```python
from build123d import *

# Parameters (mm, degrees)
SKETCH1_W           = 70.3
SKETCH1_H           = 128.3
BOSS_EXTRUDE1_DEPTH = 27.5
FILLET1_R           = 10
CUT_EXTRUDE1_START  = 35.15
CUT_EXTRUDE1_DEPTH  = 0.5
CUT_EXTRUDE2_DEPTH  = 0.5
FILLET2_R           = 10
CUT_EXTRUDE3_DEPTH  = 0.25


with BuildPart() as part:
    # Sketch1 → Boss-Extrude1 (new body)
    with BuildSketch(Plane(origin=(0, 0, 0), x_dir=(1, 0, 0), z_dir=(0, 1, 0))):
        Rectangle(SKETCH1_W, SKETCH1_H)
    extrude(amount=BOSS_EXTRUDE1_DEPTH)

    # Fillet1
    fillet1_edges = [part.edges().sort_by_distance(p)[0] for p in [
        (-35.15, 27.5, 0),
        (0, 27.5, 64.15),
        (35.15, 27.5, 0),
        (0, 0, 64.15),
        (-35.15, 0, 0),
        (0, 0, -64.15),
        (35.15, 0, 0),
        (0, 27.5, -64.15),
    ]]
    fillet(fillet1_edges, radius=FILLET1_R)

    # Sketch2 → Cut-Extrude1 (cut)
    with BuildSketch(Plane(origin=(0, 0, 0), x_dir=(0, 0, -1), z_dir=(1, 0, 0)).offset(CUT_EXTRUDE1_START)):
        with BuildLine():
            Line((48, 16.4), (53, 16.4))
            ThreePointArc((53, 16.4), (55.65, 13.75), (53, 11.1))
            Line((53, 11.1), (48, 11.1))
            ThreePointArc((48, 11.1), (45.35, 13.75), (48, 16.4))
        make_face()
        with BuildLine():
            Line((48, 15.9), (53, 15.9))
            ThreePointArc((53, 15.9), (55.15, 13.75), (53, 11.6))
            Line((53, 11.6), (48, 11.6))
            ThreePointArc((48, 11.6), (45.85, 13.75), (48, 15.9))
        make_face(mode=Mode.SUBTRACT)
    extrude(amount=-CUT_EXTRUDE1_DEPTH, mode=Mode.SUBTRACT)

    # Sketch3 → Cut-Extrude2 (cut)
    with BuildSketch(Plane(origin=(0, 27.5, 0), x_dir=(1, 0, 0), z_dir=(0, 1, 0))):
        with BuildLine():
            Line((11.275, 54.65), (20.275, 54.65))
            ThreePointArc((20.275, 54.65), (25.15, 49.775), (20.275, 44.9))
            Line((20.275, 44.9), (11.275, 44.9))
            ThreePointArc((11.275, 44.9), (6.4, 49.775), (11.275, 54.65))
        make_face()
        with BuildLine():
            Line((11.275, 54.15), (20.275, 54.15))
            ThreePointArc((20.275, 54.15), (24.65, 49.775), (20.275, 45.4))
            Line((20.275, 45.4), (11.275, 45.4))
            ThreePointArc((11.275, 45.4), (6.9, 49.775), (11.275, 54.15))
        make_face(mode=Mode.SUBTRACT)
    extrude(amount=-CUT_EXTRUDE2_DEPTH, mode=Mode.SUBTRACT)

    # Fillet2
    # the kernel refuses this fillet: 10 mm, written as the material it takes off along each edge
    with BuildSketch(Plane(origin=(25.15, 10, 54.15), x_dir=(0, 0, 1), z_dir=(1, 0, 0))) as fillet2_piece_1_section:
        Polygon((0, 0), (FILLET2_R * 1.02, 0), (FILLET2_R * 1.02, FILLET2_R * 1.02), (0, FILLET2_R * 1.02), align=None)
    fillet2_piece_1 = extrude(amount=FILLET2_R * 1.02, mode=Mode.PRIVATE)
    fillet2_piece_1 = fillet2_piece_1 - Plane(origin=(25.15, 10, 54.15), x_dir=(0, 0.7071067811865475, -0.7071067811865475), z_dir=(1, 0, 0)) * Sphere(FILLET2_R, mode=Mode.PRIVATE)
    add(fillet2_piece_1, mode=Mode.SUBTRACT)
    with BuildSketch(Plane(origin=(-25.15, 10, 54.15), x_dir=(0, 0, 1), z_dir=(-1, 0, 0))) as fillet2_piece_2_section:
        Polygon((0, 0), (FILLET2_R * 1.02, 0), (FILLET2_R * 1.02, -FILLET2_R * 1.02), (0, -FILLET2_R * 1.02), align=None)
    fillet2_piece_2 = extrude(amount=FILLET2_R * 1.02, mode=Mode.PRIVATE)
    fillet2_piece_2 = fillet2_piece_2 - Plane(origin=(-25.15, 10, 54.15), x_dir=(0, 0.7071067811865475, -0.7071067811865475), z_dir=(-1, 0, 0)) * Sphere(FILLET2_R, mode=Mode.PRIVATE)
    add(fillet2_piece_2, mode=Mode.SUBTRACT)
    with BuildSketch(Plane(origin=(25.15, 10, -54.15), x_dir=(1, 0, 0), z_dir=(0, 0, -1))) as fillet2_piece_3_section:
        Polygon((0, 0), (FILLET2_R * 1.02, 0), (FILLET2_R * 1.02, FILLET2_R * 1.02), (0, FILLET2_R * 1.02), align=None)
    fillet2_piece_3 = extrude(amount=FILLET2_R * 1.02, mode=Mode.PRIVATE)
    fillet2_piece_3 = fillet2_piece_3 - Plane(origin=(25.15, 10, -54.15), x_dir=(-0.7071067811865475, 0.7071067811865475, 0), z_dir=(0, 0, -1)) * Sphere(FILLET2_R, mode=Mode.PRIVATE)
    add(fillet2_piece_3, mode=Mode.SUBTRACT)
    with BuildSketch(Plane(origin=(-25.15, 10, -54.15), x_dir=(-1, 0, 0), z_dir=(0, 0, -1))) as fillet2_piece_4_section:
        Polygon((0, 0), (FILLET2_R * 1.02, 0), (FILLET2_R * 1.02, -FILLET2_R * 1.02), (0, -FILLET2_R * 1.02), align=None)
    fillet2_piece_4 = extrude(amount=FILLET2_R * 1.02, mode=Mode.PRIVATE)
    fillet2_piece_4 = fillet2_piece_4 - Plane(origin=(-25.15, 10, -54.15), x_dir=(0.7071067811865475, 0.7071067811865475, 0), z_dir=(0, 0, -1)) * Sphere(FILLET2_R, mode=Mode.PRIVATE)
    add(fillet2_piece_4, mode=Mode.SUBTRACT)
    with BuildSketch(Plane(origin=(-25.15, 17.5, -54.15), x_dir=(-1, 0, 0), z_dir=(0, 0, -1))) as fillet2_piece_5_section:
        Polygon((0, 0), (FILLET2_R * 1.02, 0), (FILLET2_R * 1.02, FILLET2_R * 1.02), (0, FILLET2_R * 1.02), align=None)
    fillet2_piece_5 = extrude(amount=FILLET2_R * 1.02, mode=Mode.PRIVATE)
    fillet2_piece_5 = fillet2_piece_5 - Plane(origin=(-25.15, 17.5, -54.15), x_dir=(0.7071067811865475, -0.7071067811865475, 0), z_dir=(0, 0, -1)) * Sphere(FILLET2_R, mode=Mode.PRIVATE)
    add(fillet2_piece_5, mode=Mode.SUBTRACT)
    with BuildSketch(Plane(origin=(25.15, 17.5, -54.15), x_dir=(1, 0, 0), z_dir=(0, 0, -1))) as fillet2_piece_6_section:
        Polygon((0, 0), (FILLET2_R * 1.02, 0), (FILLET2_R * 1.02, -FILLET2_R * 1.02), (0, -FILLET2_R * 1.02), align=None)
    fillet2_piece_6 = extrude(amount=FILLET2_R * 1.02, mode=Mode.PRIVATE)
    fillet2_piece_6 = fillet2_piece_6 - Plane(origin=(25.15, 17.5, -54.15), x_dir=(-0.7071067811865475, -0.7071067811865475, 0), z_dir=(0, 0, -1)) * Sphere(FILLET2_R, mode=Mode.PRIVATE)
    add(fillet2_piece_6, mode=Mode.SUBTRACT)
    with BuildSketch(Plane(origin=(-25.15, 17.5, 54.15), x_dir=(0, 0, 1), z_dir=(-1, 0, 0))) as fillet2_piece_7_section:
        Polygon((0, 0), (FILLET2_R * 1.02, 0), (FILLET2_R * 1.02, FILLET2_R * 1.02), (0, FILLET2_R * 1.02), align=None)
    fillet2_piece_7 = extrude(amount=FILLET2_R * 1.02, mode=Mode.PRIVATE)
    fillet2_piece_7 = fillet2_piece_7 - Plane(origin=(-25.15, 17.5, 54.15), x_dir=(0, -0.7071067811865475, -0.7071067811865475), z_dir=(-1, 0, 0)) * Sphere(FILLET2_R, mode=Mode.PRIVATE)
    add(fillet2_piece_7, mode=Mode.SUBTRACT)
    with BuildSketch(Plane(origin=(25.15, 17.5, 54.15), x_dir=(0, 0, 1), z_dir=(1, 0, 0))) as fillet2_piece_8_section:
        Polygon((0, 0), (FILLET2_R * 1.02, 0), (FILLET2_R * 1.02, -FILLET2_R * 1.02), (0, -FILLET2_R * 1.02), align=None)
    fillet2_piece_8 = extrude(amount=FILLET2_R * 1.02, mode=Mode.PRIVATE)
    fillet2_piece_8 = fillet2_piece_8 - Plane(origin=(25.15, 17.5, 54.15), x_dir=(0, -0.7071067811865475, -0.7071067811865475), z_dir=(1, 0, 0)) * Sphere(FILLET2_R, mode=Mode.PRIVATE)
    add(fillet2_piece_8, mode=Mode.SUBTRACT)
    with BuildSketch(Plane(origin=(-35.15, 10, -64.15), x_dir=(1, 0, 0), z_dir=(0, 1, 0)), Plane(origin=(-35.15, 10, 64.15), x_dir=(0, 0, -1), z_dir=(0, 1, 0))) as fillet2_piece_9:
        with BuildLine():
            CenterArc((FILLET2_R, -FILLET2_R), FILLET2_R, 90, 90)
            Line((0, -FILLET2_R), (0, 0))
            Line((0, 0), (FILLET2_R, 0))
        make_face()
    extrude(amount=7.5, mode=Mode.SUBTRACT)
    with BuildSketch(Plane(origin=(35.15, 10, -64.15), x_dir=(-1, 0, 0), z_dir=(0, 1, 0))) as fillet2_piece_10_section:
        with BuildLine():
            CenterArc((FILLET2_R, FILLET2_R), FILLET2_R, 180, 90)
            Line((0, FILLET2_R), (0, 0))
            Line((0, 0), (FILLET2_R, 0))
        make_face()
    fillet2_piece_10 = extrude(amount=7.5, mode=Mode.PRIVATE)
    fillet2_piece_10 = fillet2_piece_10 - Plane(origin=(30.454991339, 13.75, -53), x_dir=(0, 1, 0), z_dir=(1, 0, 0)) * Cylinder(2.15, 55, mode=Mode.PRIVATE)
    add(fillet2_piece_10, mode=Mode.SUBTRACT)
    with BuildSketch(Plane(origin=(35.15, 10, 64.15), x_dir=(0, 0, -1), z_dir=(0, 1, 0))) as fillet2_piece_11:
        with BuildLine():
            CenterArc((FILLET2_R, FILLET2_R), FILLET2_R, 180, 90)
            Line((0, FILLET2_R), (0, 0))
            Line((0, 0), (FILLET2_R, 0))
        make_face()
    extrude(amount=7.5, mode=Mode.SUBTRACT)

    # Sketch4 → Cut-Extrude3 (cut)
    with BuildSketch(Plane(origin=(0, 0, -64.15), x_dir=(-1, 0, 0), z_dir=(0, 0, -1))):
        with BuildLine():
            Line((-3.8, 15.35), (2, 15.35))
            ThreePointArc((2, 15.35), (3.6, 13.75), (2, 12.15))
            Line((2, 12.15), (-3.8, 12.15))
            ThreePointArc((-3.8, 12.15), (-5.4, 13.75), (-3.8, 15.35))
        make_face()
        with BuildLine():
            Line((-3.8, 15.1), (2, 15.1))
            ThreePointArc((2, 15.1), (3.35, 13.75), (2, 12.4))
            Line((2, 12.4), (-3.8, 12.4))
            ThreePointArc((-3.8, 12.4), (-5.15, 13.75), (-3.8, 15.1))
        make_face(mode=Mode.SUBTRACT)
    extrude(amount=-CUT_EXTRUDE3_DEPTH, mode=Mode.SUBTRACT)


solid = part.part
```
Work out the finished part from the listing and answer in its coordinate system (mm). A direction names the side the tool comes from. Coordinates: 2 decimals unless noted, no trailing zeros. Loops run counter-clockwise (first coordinate to the right, second up) from the corner with the lowest first, then second, coordinate; pieces in that order, holes last.
1) For faces 1 (the cylindrical face through (25.15, 27.25, -49.88)), 2 (the cylindrical face through (-32.3, 3.01, -0.76)), 3 (the cylindrical face through (34.9, 13.69, -45.35)), determine the directions among +Z, -Z, +X, -X, +Y, -Y from which every point of the face is accessible in a straight line to the end or side of a thin tool.
Results:
face 1: +Y
face 2: +Z, -Z, -X, -Y
face 3: +X
2) Section A-A (z = -25) is taken. Give the vertices of the cut face in (x, y), plus the area to 3 significant figures.
Results:
outline: (-35.15, 10) arc R10 ccw to (-25.15, 0) - (25.15, 0) arc R10 ccw to (35.15, 10) - (35.15, 17.5) arc R10 ccw to (25.15, 27.5) - (-25.15, 27.5) arc R10 ccw to (-35.15, 17.5) - close
area: 1,850 mm2
3) Consider probe 1 along X at (y, z) = (9.25, -15); probe 2 along Z at (x, y) = (21, 9.25); probe 3 along Y at (x, z) = (25.5, 28.5). Determine where each line is inside the solid, lowest interval first.
Results:
probe 1: x = -35.12 to 35.12
probe 2: z = -64.12 to 64.12
probe 3: y = 0.01 to 27.49
4) Section B-B (y = 2) is taken. Give the vertices of the cut face in (x, z), plus the area to 3 significant figures.
Results:
outline: (-31.15, -54.15) arc R6 ccw to (-25.15, -60.15) - (25.15, -60.15) arc R6 ccw to (31.15, -54.15) - (31.15, 54.15) arc R6 ccw to (25.15, 60.15) - (-25.15, 60.15) arc R6 ccw to (-31.15, 54.15) - close
area: 7,460 mm2
5) A flat-ended cylindrical pin translates along its axis: pin 1 (4 mm diameter, centred on y = 24, z = -21.5, fed in from -X). Find the tip coordinate at first contact, or state that the pin passes through.
Results:
pin 1: stops at x = -34.08
6) For a pull along Z with two mould halves and no side action, classify faces 4 (the cylindrical face through (0.35, 24.49, 61.3)), 5 (the flat face through (34.65, 16.1, -50.1)), 6 (the cylindrical face through (32.3, 24.49, -0.76)), 7 (the cylindrical face through (34.85, 13.81, -55.65)) as +Z half, -Z half, draft (parallel to the pull), parting line (faces both ways), or undercut.
Results:
face 4: +Z half
face 5: undercut
face 6: draft
face 7: undercut
